Here's how the part is built. I have some questions about the finished solid (model axes, mm). A direction names the side the tool comes from. Coordinates: 2 decimals unless noted, no trailing zeros. Write each loop counter-clockwise with the first axis right and the second up, starting at its lowest first coordinate (ties: lowest second). Pieces come first, ordered by that corner, then holes.
Autodesk Inventor part; units mm, degrees
ref_plane "YZ Plane" through (0, 0, 0) normal (1, 0, 0) x (0, 1, 0)
ref_plane "XZ Plane" through (0, 0, 0) normal (0, 1, 0) x (-1, 0, 0)
ref_plane "XY Plane" through (0, 0, 0) normal (0, 0, 1) x (1, 0, 0)
sketch "Sketch1" plane through (0, 0, 0) normal (0, 1, 0) x (-1, 0, 0)
  circle A0 centre (0, 0) radius 13.97
  dimension "d0" = 27.94
extrude "Extrusion1" add sketch "Sketch1" along normal blind 2.54
sketch "Sketch2" plane through (0, 2.54, 0) normal (0, 1, 0) x (1, 0, 0)
  circle A0 centre (0, 0) radius 13.97
  circle A1 centre (0, 0) radius 11.7475
  dimension "d3" = 23.495
extrude "Extrusion2" add sketch "Sketch2" along normal blind 7.62
sketch "Sketch3" plane through (0, 2.54, 0) normal (0, 1, 0) x (1, 0, 0)
  circle A0 centre (0, 0) radius 6.35
  dimension "d6" = 12.7
extrude "Extrusion3" add sketch "Sketch3" along normal blind 7.62
chamfer "Chamfer1" distance 2.54 distance2 7.62 1 edges at (-6.35, 10.16, 0) measured on face at (-1.8127, 10.16, 0.4771)
sketch "Sketch4" plane through (0, 0, 0) normal (0, -1, 0) x (1, 0, 0)
  circle A0 centre (0, 0) radius 3.81
  dimension "d12" = 7.62
extrude "Extrusion4" add sketch "Sketch4" along normal blind 17.78
sketch "Sketch5" plane through (0, -17.78, 0) normal (0, -1, 0) x (1, 0, 0)
  circle A0 centre (0, 0) radius 1.911
  circle A1 centre (0, 0) radius 3.81
  circle A2 centre (0, 0) radius 1.911
extrude "Extrusion5" cut sketch "Sketch5" against normal blind 17.78
sketch "Sketch6" plane through (0, -17.78, 0) normal (0, -1, 0) x (1, 0, 0)
  circle A0 centre (0, 0) radius 3.81
  dimension "d17" = 7.62
extrude "Extrusion6" add sketch "Sketch6" along normal blind 12.7
properties part number "cap_20mL"
1) Will these pins go through, and if not, where does the flat tip stop? pin 1 (8 mm diameter, centred on x = 4.5, y = -9, fed in from -Z); pin 2 (2 mm diameter, centred on x = 1.5, y = -4.5, fed in from +Z); pin 3 (1.5 mm diameter, centred on x = 1, z = 8, fed in from +Y).
Values follow:
pin 1: stops at z = -1.84
pin 2: stops at z = 1.84
pin 3: stops at y = 2.54
2) We'd pull the mould along Z, two halves only. Please class faces 4 (the face through (-2, -17.78, -1)), 5 (the face through (-0.414, -9.014, -1.866)), 6 (the face through (-2.547, 6.297, -11.468)): pulls with the +Z half, pulls with the -Z half, needs draft (parallel to the pull), parting line crosses it, or undercut.
Values follow:
face 4: needs draft
face 5: parting line crosses it
face 6: undercut
3) Imagine slicing it at A-A on y = -9. Please give me the cut outline in (x, z), then the cut area to 3 significant figures.
Values follow:
outline: circle Ø3.82 at (0, 0)
area: 11.5 mm2
4) Imagine slicing it at B-B on y = 6. Please give me the cut outline in (x, z) (1 decimal), then the cut area to 3 significant figures.
Values follow:
outline: circle Ø27.9 at (0, 0); circle Ø10.4 at (0, 0); hole circle Ø23.5 at (0, 0)
area: 264 mm2
5) I need wall thicknesses on probe 1 along Y at (x, z) = (1.5, 3); probe 2 along X at (y, z) = (5.5, -1.5); probe 3 along X at (y, z) = (4.5, 0). Which ranges of each line are inside material? Lowest first, please.
Values follow:
probe 1: y = -30.48 to -17.78, 0 to 10.16
probe 2: x = -13.89 to -11.65, -5.15 to 5.15, 11.65 to 13.89
probe 3: x = -13.97 to -11.75, -5.7 to 5.7, 11.75 to 13.97
6) On a 3-axis mill with a long thin cutter (end or side, diameter ignored), from which of +Z, -Z, +X, -X, +Y, -Y can I reach the whole of each face in a straight line? I mean faces 1 (the face through (-0.83, -24.04, 3.72)), 2 (the face through (-5, 2.54, -5)), 3 (the face through (0.92, 5.01, 13.94)). Say none if no direction works.
Values follow:
face 1: -Y
face 2: +Y
face 3: +Y, -Y
7) Imagine slicing it at C-C on y = -27.5. Please give me the cut outline in (x, z), then the cut area to 3 significant figures.
Values follow:
outline: circle Ø7.62 at (0, 0)
area: 45.6 mm2
